from build123d import *

# Parameters (mm, degrees)
F0_W     = 152.4
F0_H     = 152.4
F1_DEPTH = 152.4
F2_T     = -5.08
F3_R     = 2.53999


# Not quite as in the source:
# - a fillet or chamfer is up to 0.001 mm smaller than in the source, because OpenCascade refuses the exact size


with BuildPart() as f1:
    # F0 (on Top) → F1 (new body)
    with BuildSketch(Plane.XY):
        Rectangle(F0_W, F0_H)
    extrude(amount=F1_DEPTH)

    # F2
    f2_openings = [f1.faces().sort_by_distance(p)[0] for p in [
        (0, 0, 152.4),
    ]]
    offset(amount=F2_T, openings=f2_openings)

    # F3 (radius 2.54 in the source; OpenCascade refuses exactly that, so slightly less here)
    f3_edges = [f1.edges().sort_by_distance(p)[0] for p in [
        (76.2, 0, 152.4),
        (0, 76.2, 152.4),
        (-76.2, 0, 152.4),
        (0, -76.2, 152.4),
        (71.12, 0, 152.4),
        (0, -71.12, 152.4),
        (-71.12, 0, 152.4),
        (0, 71.12, 152.4),
        (76.2, 76.2, 76.2),
        (-76.2, 76.2, 76.2),
        (0, 76.2, 0),
        (71.12, 0, 5.08),
        (0, 71.12, 5.08),
        (-71.12, 0, 5.08),
        (0, -71.12, 5.08),
        (-71.12, -71.12, 78.74),
        (-71.12, 71.12, 78.74),
        (71.12, -71.12, 78.74),
        (71.12, 71.12, 78.74),
        (-76.2, -76.2, 76.2),
        (-76.2, 0, 0),
        (76.2, -76.2, 76.2),
        (0, -76.2, 0),
        (76.2, 0, 0),
    ]]
    fillet(f3_edges, radius=F3_R)


solid = f1.part
Build history of the part. All positions in model axes, mm. A direction names the side the tool comes from. Coordinates: 2 decimals unless noted, no trailing zeros. Order: outer loops, then holes, each group sorted by start corner. A loop starts at its lowest first (then second) coordinate and runs counter-clockwise, first axis right, second up. Notation, with made-up numbers: (-1.75, -24) -> (26.25, -24) arc R20 ccw to (26.25, -17) -> close; hole circle Ø4 at (-24, 63). An arc over 180 degrees is marked (long way). One line per item, written item: value.
(1) Slice it at A-A, the plane z = 105. List the corners of the cut face in (x, y).
Checked values:
outline: (-76.2, -73.66) arc R2.54 ccw to (-73.66, -76.2) -> (73.66, -76.2) arc R2.54 ccw to (76.2, -73.66) -> (76.2, 73.66) arc R2.54 ccw to (73.66, 76.2) -> (-73.66, 76.2) arc R2.54 ccw to (-76.2, 73.66) -> close; hole (-71.12, -68.58) arc R2.54 ccw to (-68.58, -71.12) -> (68.58, -71.12) arc R2.54 ccw to (71.12, -68.58) -> (71.12, 68.58) arc R2.54 ccw to (68.58, 71.12) -> (-68.58, 71.12) arc R2.54 ccw to (-71.12, 68.58) -> close
(2) Tool access for faces 4 (the flat face through (-1, -71.12, 78)), 5 (the flat face through (-1, -76.2, 75)): list every direction of +Z, -Z, +X, -X, +Y, -Y with a clear straight run to the whole face (end or side of a thin tool).
Checked values:
face 4: +Z
face 5: +Z, -Z, +X, -X, -Y
(3) Mould opens along X. For faces 1 (the flat face through (76.2, -1, 75)), 2 (the flat face through (-76.2, -1, 75)), 3 (the flat face through (-1, 1, 5.08)) say: pulls with the +X half, pulls with the -X half, needs draft (parallel to the pull), parting line crosses it, or undercut.
Checked values:
face 1: pulls with the +X half
face 2: pulls with the -X half
face 3: undercut
(4) Drop flat-ended pins along their axis: pin 1 Ø5 at (x, y) = (2.5, -10) entering from -Z; pin 2 Ø12 at (x, y) = (16.5, -41) entering from +Z. Give the stop position or say it passes through.
Checked values:
pin 1: z = 0
pin 2: z = 5.08
(5) Probe line 1 (X direction, y = 62, z = 29.5); line 2 (Z direction, x = 44, y = 28.5). List the from-to ranges inside material, lowest first. Write a range as [from, to].
Checked values:
line 1: [-76.2, -71.12], [71.12, 76.2]
line 2: [0, 5.08]
